Verification items for the finished model (mm, model axes). Round coordinates to 2 decimals unless told otherwise and drop trailing zeros. Write each loop counter-clockwise with the first axis right and the second up, starting at its lowest first coordinate (ties: lowest second). Pieces come first, ordered by that corner, then holes.
from build123d import *

# Parameters (mm, degrees)
BOSS_EXTRU_1_DEPTH      = 1.5
ESQUISSE2_R             = 1.5
ENL_V_MAT_EXTRU_1_DEPTH = 342.283606404
CONG_1_R                = 5
CONG_2_R                = 15
ESQUISSE3_R             = 1.5
ENL_V_MAT_EXTRU_2_DEPTH = 342.283606404


with BuildPart() as part:
    # Esquisse1 → Boss.-Extru.1 (new body)
    with BuildSketch(Plane.XY):
        Polygon((185.25, 171.5), (203.25, 190), (255.5, 190), (283.5, 168.124002458), (283.5, 0), (0, 0), (0, 171.5), align=None)
    extrude(amount=BOSS_EXTRU_1_DEPTH)

    # Esquisse2 → Enlèv. mat.-Extru.1 (cut, through all)
    with BuildSketch(Plane.XY.offset(1.5)):
        with Locations((261.75, 5)):
            Circle(ESQUISSE2_R)
        with Locations((181.75, 5)):
            Circle(ESQUISSE2_R)
        with Locations((101.75, 5)):
            Circle(ESQUISSE2_R)
        with Locations((21.75, 5)):
            Circle(ESQUISSE2_R)
        with Locations((7.5, 75)):
            Circle(ESQUISSE2_R)
        with Locations((7.5, 150)):
            Circle(ESQUISSE2_R)
        with Locations((87.75, 164)):
            Circle(ESQUISSE2_R)
        with Locations((185.25, 167.5)):
            Circle(ESQUISSE2_R)
        with Locations((205.25, 186)):
            Circle(ESQUISSE2_R)
        with Locations((230, 165)):
            Circle(ESQUISSE2_R)
        with Locations((250, 185)):
            Circle(ESQUISSE2_R)
        with Locations((273.5, 165)):
            Circle(ESQUISSE2_R)
    extrude(amount=-ENL_V_MAT_EXTRU_1_DEPTH, mode=Mode.SUBTRACT)

    # Congé1
    cong_1_edges = [part.edges().sort_by_distance(p)[0] for p in [
        (185.25, 171.5, 0.75),
        (203.25, 190, 0.75),
        (255.5, 190, 0.75),
        (283.5, 168.124002458, 0.75),
    ]]
    fillet(cong_1_edges, radius=CONG_1_R)

    # Congé2
    cong_2_edges = [part.edges().sort_by_distance(p)[0] for p in [
        (0, 171.5, 0.75),
    ]]
    fillet(cong_2_edges, radius=CONG_2_R)

    # Esquisse3 → Enlèv. mat.-Extru.2 (cut, through all)
    with BuildSketch(Plane.XY.offset(1.5)):
        with Locations((198.5, 131.5)):
            Circle(ESQUISSE3_R)
        with Locations((258.5, 131.5)):
            Circle(ESQUISSE3_R)
    extrude(amount=-ENL_V_MAT_EXTRU_2_DEPTH, mode=Mode.SUBTRACT)


solid = part.part
Q1. Sectioned sample at B-B (x = 50). Enter the section's corners in (y, z).
Recorded:
outline: (0, 0) - (171.5, 0) - (171.5, 1.5) - (0, 1.5) - close
Q2. Material ranges on line 1 along X through (y, z) = (164, 0.7); line 2 along X through (y, z) = (186, 0.95); line 3 along Y through (x, z) = (7.5, 1), recorded low to high.
Recorded:
line 1: x = 2.01 to 86.25, 89.25 to 228.88, 231.12 to 272.38, 274.62 to 283.5
line 2: x = 199.36 to 203.75, 206.75 to 248.88, 251.12 to 260.62
line 3: y = 0 to 73.5, 76.5 to 148.5, 151.5 to 169.49
Q3. Sectioned sample at A-A (z = 0.3). Give the number of separate pieces and of enclosed holes in the cut face, plus the area to 3 significant figures.
Recorded:
separate pieces: 1
enclosed holes: 14
area: 49,800 mm2
